Input: part model. Units: mm. Frame: model coordinates. Face numbers are marked on the shaded views. A direction names the side the tool comes from. Round coordinates to 2 decimals unless told otherwise and drop trailing zeros. Write each loop counter-clockwise with the first axis right and the second up, starting at its lowest first coordinate (ties: lowest second). Pieces come first, ordered by that corner, then holes. Notation, with made-up numbers: (49.5, 40) -> (88.5, 40) arc R13 ccw to (88.5, 61) -> close; hole circle Ø10 at (89.5, -26.5). An arc over 180 degrees is marked (long way). Use CSV: the item, a comma, the result in double quotes.
Autodesk Inventor part; units mm, degrees
ref_plane "YZ Plane" through (0, 0, 0) normal (1, 0, 0) x (0, 1, 0)
ref_plane "XZ Plane" through (0, 0, 0) normal (0, 1, 0) x (-1, 0, 0)
ref_plane "XY Plane" through (0, 0, 0) normal (0, 0, 1) x (1, 0, 0)
sketch "Sketch1" plane through (0, 0, 0) normal (1, 0, 0) x (0, 1, 0)
  line L0 (46, 10) -> (-10, 10)
  line L1 (46, -90) -> (-10, -90)
  line L2 (46, 10) -> (46, -90)
  line L3 (-10, 10) -> (-10, -90)
  point P0 (0, 0)
  dimension "d4" = 100
extrude "Extrusion1" add sketch "Sketch1" along normal blind 10
sketch "Sketch2" plane through (10, 0, 0) normal (1, 0, 0) x (0, 0, -1)
  line L0 (0, 36) -> (80, 36)
  line L1 (80, 36) -> (80, 0)
  line L2 (80, 0) -> (0, 0)
  line L3 (0, 0) -> (0, 36)
  line L4 (90, 46) -> (-10, 46)
  line L5 (-10, -10) -> (90, -10)
  line L6 (-10, 46) -> (-10, -10)
  line L7 (90, -10) -> (90, 46)
  point P0 (0, 0)
  dimension "d9" = 80
  dimension "d10" = 36
  dimension "d11" = 10
  dimension "d12" = 10
  dimension "d13" = 10
  dimension "d14" = 10
extrude "Extrusion2" cut sketch "Sketch2" against normal blind 2 contours L0 L1 L2 L3
sketch "Sketch3" plane through (10, 0, 0) normal (0, 1, 0) x (1, 0, 0)
  circle A0 centre (-2.8864, 52.3034) radius 1.5
  circle A1 centre (-2.8864, 32.3034) radius 1.5
  line L0 (0, 80) -> (-2, 80)
  line L1 (0, 0) -> (-2, 0)
  point P0 (-10, 0)
  dimension "d17" = 3
  dimension "d18" = 3
  dimension "d19" = 20
  dimension "d20" = 27.6966
  dimension "d21" = 32.3034
extrude "Extrusion3" cut sketch "Sketch3" against normal through all
sketch "Sketch4" plane through (8, 0, 0) normal (1, 0, 0) x (0, 0, -1)
  circle A0 centre (36.6715, 5.3743) radius 2.5605
  point P0 (0, 0)
extrude "Extrusion4" cut sketch "Sketch4" against normal through all
sketch "Sketch5" plane through (0, -10, -90) normal (0, -1, 0) x (1, 0, 0)
  line L0 (8, 10) -> (8, 90)
  circle A0 centre (8, 90) radius 4
  line L1 (10, 10) -> (8, 10)
  circle A1 centre (8, 10) radius 4
  point P0 (0, 90)
  dimension "d26" = 8
  dimension "d27" = 8
extrude "Extrusion5" add sketch "Sketch5" along normal blind 40
sketch "Sketch6" plane through (0, -10, -90) normal (0, -1, 0) x (1, 0, 0)
  point P0 (0, 90)
sketch "Sketch8" plane through (0, -10, -90) normal (0, -1, 0) x (1, 0, 0)
  point P0 (0, 90)
sketch "Sketch9" plane through (10, 0, 0) normal (1, 0, 0) x (0, 0, -1)
  point P0 (0, 0)
sketch "Sketch10" plane through (0, 0, 0) normal (-1, 0, 0) x (0, 0, 1)
  line L0 (-78.8319, 36.3964) -> (1.1681, 36.3964)
  line L1 (1.1681, 36.3964) -> (1.1681, 0.3964)
  line L2 (1.1681, 0.3964) -> (-78.8319, 0.3964)
  line L3 (-78.8319, 0.3964) -> (-78.8319, 36.3964)
  point P0 (0, 0)
  dimension "d34" = 80
  dimension "d35" = 36
extrude "Extrusion7" cut sketch "Sketch10" against normal blind 2
properties part number "upper part edited" material "Polyethylene, High Density"
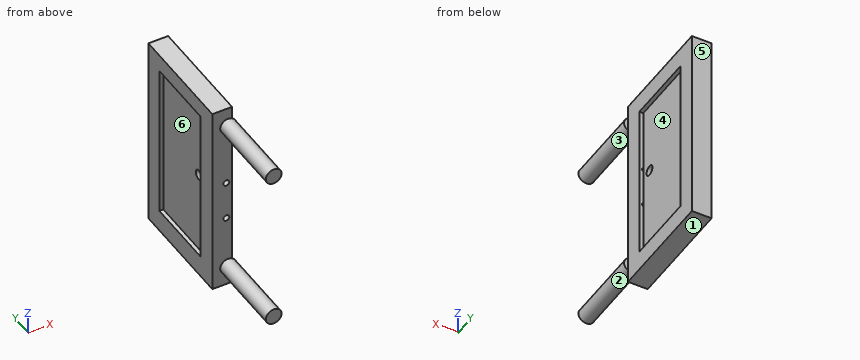
Item 1: Set-up query: the marked faces 1 and 2. Return all of +Z, -Z, +X, -X, +Y, -Y with unobstructed straight access to the full face (end or side cutting, diameter ignored); none if empty.
Worked answers:
face 1,"-Z, +X, -X, +Y, -Y"
face 2,"-Y"
Item 2: Line query: line 1 (Y direction, x = 9, z = -75); line 2 (Z direction, x = 1.75, y = 36); line 3 (Z direction, x = 6, y = -29). Output: solid intervals per line, ascending.
Worked answers:
line 1,"y = -10 to 0, 36 to 46"
line 2,"z = -90 to -78.83, 1.17 to 10"
line 3,"z = -83.46 to -76.54, -3.46 to 3.46"
Item 3: Section query B-B on z = -63. Return the cut outline in (x, y), plus the area to 3 significant figures.
Worked answers:
outline,"(0, -10) -> (10, -10) -> (10, 0) -> (8, 0) -> (8, 36) -> (10, 36) -> (10, 46) -> (0, 46) -> (0, 36.4) -> (2, 36.4) -> (2, 0.4) -> (0, 0.4) -> close"
area,"416 mm²"
Item 4: Pull-direction query (Y, two-part tool) for the marked faces 3, 4, 5 and 6; classes: +Y half, -Y half, draft (parallel to the pull), parting line (faces both ways), or undercut.
Worked answers:
face 3,"draft"
face 4,"undercut"
face 5,"+Y half"
face 6,"undercut"
Item 5: First-contact query: pin 1 Ø6 at (x, z) = (3.5, -25) entering from -Y; pin 2 Ø1.9 at (x, z) = (7, -52.5) entering from -Y; pin 3 Ø2 at (y, z) = (19, -37.5) entering from -X. Flat tips, straight axial feed; report the tip coordinate or a pass-through.
Worked answers:
pin 1,"stops at y = -10"
pin 2,"stops at y = 0"
pin 3,"stops at x = 2"
Item 6: Section query A-A on y = 14. Return the cut outline in (x, z).
Worked answers:
outline,"(0, -90) -> (10, -90) -> (10, -80) -> (8, -80) -> (8, 0) -> (10, 0) -> (10, 10) -> (0, 10) -> (0, 1.17) -> (2, 1.17) -> (2, -78.83) -> (0, -78.83) -> close"
